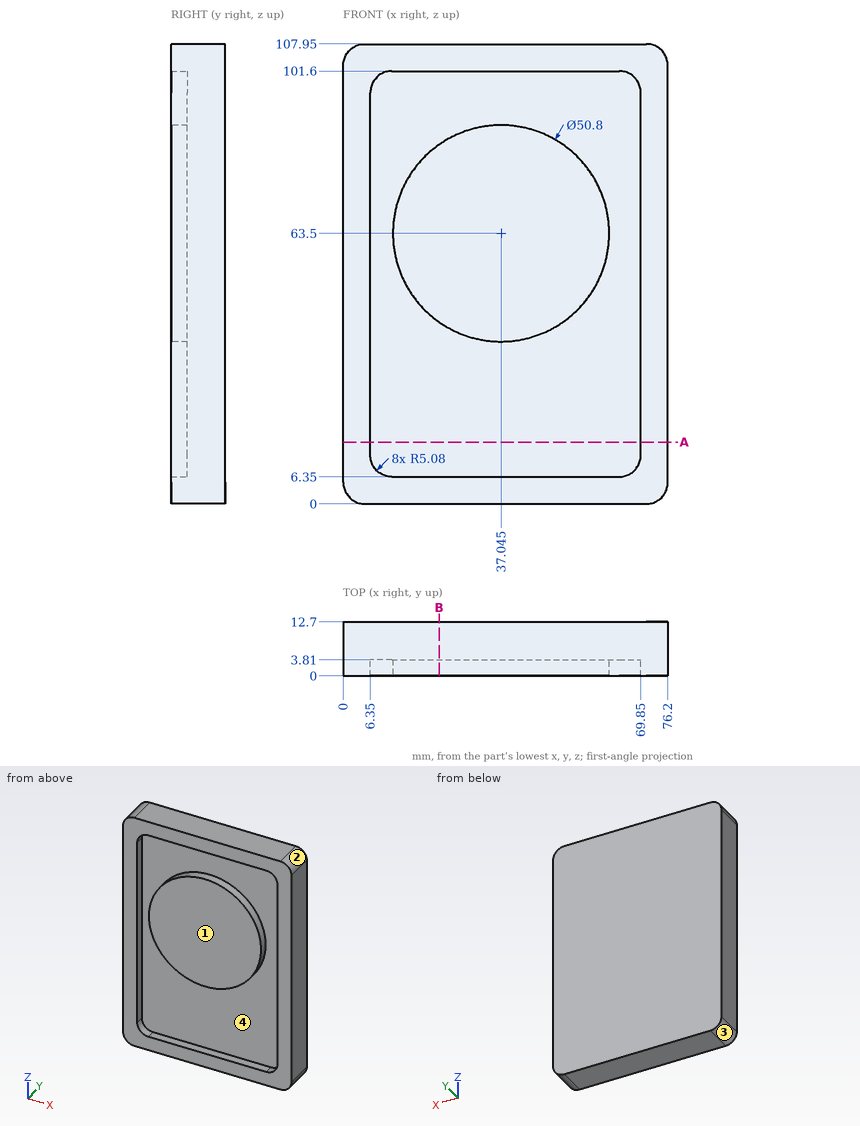
Answer from the drawing. Dimensions are ordinates in mm from the lowest x, y and z of the part. Give positions to 0.01 mm unless a question says otherwise; leave off trailing zeros. Order: outer loops, then holes, each group sorted by start corner. A loop starts at its lowest first (then second) coordinate and runs counter-clockwise, first axis right, second up. Notation, with made-up numbers: (48, 61) -> (61, 61) arc R8 cw to (61, 67) -> close; hole circle Ø8 at (40.5, -37.75). An arc over 180 degrees is marked (long way). Answer as a JSON object with one key per item and string values. Group by question number.
1. Section B-B on x = 22.5 is taken. Determine the outline of the cut face in (y, z), plus the area to 3 significant figures.
2. Section A-A on z = 14.5 is taken. Determine the outline of the cut face in (x, y).
3. The mould has two halves that part along Z. Classify the marked faces 1, 2, 3 and 4: released by +Z, released by -Z, zero draft, split by the parting line, or undercut.
4. A flat-ended cylindrical pin translates along its axis: pin 1 Ø4 at (x, z) = (62.5, 88) entering from -Y. Find the tip coordinate at first contact, or state that the pin passes through.
5. Consider line 1 along X through (y, z) = (1.25, 29); line 2 along Z through (x, y) = (54, 2.75); line 3 along Y through (x, z) = (52.5, 6.5). Determine where each line is inside the solid, lowest interval first. Write a range as [from, to].
Result sheet:
{
 "1": {"outline": "(0, 0) -> (12.7, 0) -> (12.7, 107.95) -> (0, 107.95) -> (0, 101.6) -> (3.81, 101.6) -> (3.81, 84.32) -> (0, 84.32) -> (0, 42.68) -> (3.81, 42.68) -> (3.81, 6.35) -> (0, 6.35) -> close", "area": "1,170 mm^2"},
 "2": {"outline": "(0, 0) -> (6.35, 0) -> (6.35, 3.81) -> (69.85, 3.81) -> (69.85, 0) -> (76.2, 0) -> (76.2, 12.7) -> (0, 12.7) -> close"},
 "3": {"face 1": "zero draft", "face 2": "released by +Z", "face 3": "released by -Z", "face 4": "undercut"},
 "4": {"pin 1": "stops at y = 3.81"},
 "5": {"line 1": "x = [0, 6.35], [69.85, 76.2]", "line 2": "z = [0, 6.35], [44.59, 82.41], [101.6, 107.95]", "line 3": "y = [3.81, 12.7]"}
}
